Verification items for the finished model (mm, model axes). A direction names the side the tool comes from. Give positions to 0.01 mm unless a question says otherwise; leave off trailing zeros. Order: outer loops, then holes, each group sorted by start corner. A loop starts at its lowest first (then second) coordinate and runs counter-clockwise, first axis right, second up. Notation, with made-up numbers: (-16.75, -0.75) - (0.25, -0.75) arc R15 cw to (0.25, 23.25) - close; hole circle Ø4 at (61.25, -22). An arc over 180 degrees is marked (long way). Answer as a JSON object with one key per item and string values. Group by question number.
(1) Section check C-C (x = 101.5). Record the boundary of the cut face in (y, z) (1 decimal).
(2) Mould release check, pull along X, two halves, no side actions. Record for faces 1 (the face through (-2, 1, 0)), 2 (the face through (125.72, 17.09, 1.61)): +X half, -X half, draft (parallel to the pull), parting line (faces both ways), or undercut.
(3) Section check A-A (z = 2). Count the separate pieces of the cut face and the enclosed holes in it, then the cut area to 3 significant figures.
(4) Section check B-B (x = -97.75). Record the boundary of the cut face in (y, z) (1 decimal).
(5) Depth check by flat-ended pin: pin 1 Ø3.5 at (x, y) = (-109.75, -9.76) entering from +Z. Enter the tip coordinate at first touch or a pass-through.
(6) Access from +Z, -Z, +X, -X, +Y, -Y to the whole of each face (thin tool, end or side, straight path). Record for faces 3 (the face through (118.664, -30.857, 1.61)), 4 (the face through (97.607, -3.264, 1.565)).
(7) Thickness scan on line 1 (X direction, y = -1, z = 2.15); line 2 (X direction, y = -16, z = 2.6); line 3 (Y direction, x = -109.75, z = 1.1). Record the ranges inside material, lowest first.
```python
from build123d import *

# Parameters (mm, degrees)
SKETCH1_W            = 299.7
SKETCH1_H            = 76.075
BOSS_EXTRUDE1_DEPTH  = 3.175
CUT_EXTRUDE4_DEPTH   = 155.634907221
SKETCH3_R            = 6.5
CUT_EXTRUDE5_DEPTH   = 155.634907221
M4_CLEARANCE_HOLE1_D = 4.5


with BuildPart() as part:
    # Sketch1 → Boss-Extrude1 (new body)
    with BuildSketch(Plane.XY):
        Rectangle(SKETCH1_W, SKETCH1_H)
    extrude(amount=BOSS_EXTRUDE1_DEPTH)

    # Sketch8 → Cut-Extrude4 (cut, through all)
    with BuildSketch(Plane.XY.offset(3.175)):
        with BuildLine():
            Line((122.1609, 18.5125), (122.2247, 18.5125))
            ThreePointArc((122.2247, 18.5125), (125.760233906, 17.048033906), (127.2247, 13.5125))
            Line((127.2247, 13.5125), (127.2247, -27.282435401))
            ThreePointArc((127.2247, -27.282435401), (125.760233906, -30.817969307), (122.2247, -32.282435401))
            Line((122.2247, -32.282435401), (122.1609, -32.282435401))
            ThreePointArc((122.1609, -32.282435401), (118.625366094, -30.817969307), (117.1609, -27.282435401))
            Line((117.1609, -27.282435401), (117.1609, 13.5125))
            ThreePointArc((117.1609, 13.5125), (118.625366094, 17.048033906), (122.1609, 18.5125))
        make_face()
    cut_extrude4 = extrude(amount=-CUT_EXTRUDE4_DEPTH, mode=Mode.SUBTRACT)

    # Mirror3: Cut-Extrude4 across plane
    add(cut_extrude4.mirror(Plane(origin=(0, 0, 0), x_dir=(0, 0, 1), z_dir=(1, 0, 0))), mode=Mode.SUBTRACT)

    # Sketch3 → Cut-Extrude5 (cut, through all)
    with BuildSketch(Plane(origin=(0, 0, 0), x_dir=(-1, 0, 0), z_dir=(0, 0, -1))):
        with Locations((-97.75, -9.7625)):
            Circle(SKETCH3_R)
        with BuildLine():
            Line((-104.25, -38.0375), (-91.25, -38.0375))
            Line((-91.25, -38.0375), (-91.25, -9.7625))
            ThreePointArc((-91.25, -9.7625), (-97.75, -16.2625), (-104.25, -9.7625))
            Line((-104.25, -9.7625), (-104.25, -38.0375))
        make_face()
        with Locations((97.75, -9.7625)):
            Circle(SKETCH3_R)
        with BuildLine():
            Line((91.25, -38.0375), (104.25, -38.0375))
            Line((104.25, -38.0375), (104.25, -9.7625))
            ThreePointArc((104.25, -9.7625), (97.75, -16.2625), (91.25, -9.7625))
            Line((91.25, -9.7625), (91.25, -38.0375))
        make_face()
    extrude(amount=-CUT_EXTRUDE5_DEPTH, mode=Mode.SUBTRACT)

    # M4 Clearance Hole1 (through all)
    with Locations(Plane(origin=(0, 0, 0), x_dir=(-1, 0, 0), z_dir=(0, 0, -1))):
        with Locations((-85.75, -9.7625), (-109.75, -9.7625), (109.75, -9.7625), (85.75, -9.7625)):
            Hole(M4_CLEARANCE_HOLE1_D / 2)


solid = part.part
```
Solutions:
{
 "1": {"outline": "(-4.5, 0) - (38, 0) - (38, 3.2) - (-4.5, 3.2) - close"},
 "2": {"face 1": "draft", "face 2": "undercut"},
 "3": {"separate pieces": "1", "enclosed holes": "6", "area": "20,900 mm2"},
 "4": {"outline": "(-3.3, 0) - (38, 0) - (38, 3.2) - (-3.3, 3.2) - close"},
 "5": {"pin 1": "passes through"},
 "6": {"face 3": "+Z, -Z", "face 4": "+Z, -Z, -Y"},
 "7": {"line 1": "x = -149.85 to -127.22, -117.16 to 117.16, 127.22 to 149.85", "line 2": "x = -149.85 to -127.22, -117.16 to -104.25, -91.25 to 91.25, 104.25 to 117.16, 127.22 to 149.85", "line 3": "y = -38.04 to -12.01, -7.51 to 38.04"}
}
